```python
from build123d import *

# Parameters (mm, degrees)
F1_DEPTH = 30.1625
F2_DEPTH = 11.1633
F4_DEPTH = 19.05
F5_DEPTH = 19.05
F6_R     = 7.874
F7_R     = 5.08
F8_R     = 6.35
F9_DEPTH = 22.353


with BuildPart() as f1:
    # F0 (on Front) → F1 (new body, symmetric)
    with BuildSketch(Plane.XZ):
        Polygon((97.8408, -22.352), (117.2485877871, -22.352), (117.2485877871, 0), (91.8464, 0), align=None)
        Polygon((91.8464, -22.352), (91.8464, 0), (85.852, 0), align=None)
        Polygon((64.8810639977, -22.352), (91.8464, -22.352), (85.852, 0), (43.9732931554, 0), align=None)
        with BuildLine():
            Line((0, -22.352), (64.8810639977, -22.352))
            Line((64.8810639977, -22.352), (43.9732931554, 0))
            Line((43.9732931554, 0), (22.352, 0))
            ThreePointArc((22.352, 0), (15.8052507731, -15.8052507731), (0, -22.352))
        make_face()
        with BuildLine():
            ThreePointArc((22.352, 0), (-15.8052507731, 15.8052507731), (0, -22.352))
            Line((0, -22.352), (0, -12.7))
            ThreePointArc((0, -12.7), (-8.9802561211, 8.9802561211), (12.7, 0))
            Line((12.7, 0), (22.352, 0))
        make_face()
        Polygon((91.8464, -22.352), (97.8408, -22.352), (91.8464, 0), align=None)
        Polygon((194.2084, -22.352), (194.2084, 0), (150.0886, 0), (131.0386, 0), (117.2485877871, 0), (117.2485877871, -22.352), align=None)
        with BuildLine():
            Line((0, -12.7), (0, -22.352))
            ThreePointArc((0, -22.352), (15.8052507731, -15.8052507731), (22.352, 0))
            Line((22.352, 0), (12.7, 0))
            ThreePointArc((12.7, 0), (8.9802561211, -8.9802561211), (0, -12.7))
        make_face()
    extrude(amount=F1_DEPTH, both=True)

    # F0 (on Front) → F2 (cut, symmetric)
    with BuildSketch(Plane.XZ):
        with BuildLine():
            ThreePointArc((22.352, 0), (-15.8052507731, 15.8052507731), (0, -22.352))
            Line((0, -22.352), (0, -12.7))
            ThreePointArc((0, -12.7), (-8.9802561211, 8.9802561211), (12.7, 0))
            Line((12.7, 0), (22.352, 0))
        make_face()
        with BuildLine():
            Line((0, -12.7), (0, -22.352))
            ThreePointArc((0, -22.352), (15.8052507731, -15.8052507731), (22.352, 0))
            Line((22.352, 0), (12.7, 0))
            ThreePointArc((12.7, 0), (8.9802561211, -8.9802561211), (0, -12.7))
        make_face()
    extrude(amount=F2_DEPTH, both=True, mode=Mode.SUBTRACT)

    # F3 (on face) → F4 (cut)
    with BuildSketch(Plane.XZ.offset(30.1625)):
        Polygon((117.2485877871, -22.352), (117.2485877871, 0), (85.852, 0), (91.8464, -22.352), align=None)
    extrude(amount=-F4_DEPTH, mode=Mode.SUBTRACT)

    # F3 (on face) → F5 (join)
    with BuildSketch(Plane.XZ.offset(30.1625)):
        with BuildLine():
            ThreePointArc((131.0386, 34.798), (127.4654323074, 16.0825969798), (117.2485877871, 0))
            Line((117.2485877871, 0), (150.0886, 0))
            Line((150.0886, 0), (150.0886, 34.798))
            Line((150.0886, 34.798), (131.0386, 34.798))
        make_face()
    extrude(amount=-F5_DEPTH)

    # F6
    f6_edges = [f1.edges().sort_by_distance(p)[0] for p in [
        (194.2084, 0, 0),
    ]]
    fillet(f6_edges, radius=F6_R)

    # F7
    f7_edges = [f1.edges().sort_by_distance(p)[0] for p in [
        (150.0886, -20.6375, 34.798),
        (150.0886, -20.6375, 0),
        (22.352, 20.6629, 0),
        (22.352, -20.6629, 0),
    ]]
    fillet(f7_edges, radius=F7_R)

    # F8 (on face) → F9 (cut, through all)
    with BuildSketch(Plane.XY):
        with Locations((155.3464, 7.8105)):
            Circle(F8_R)
    extrude(amount=-F9_DEPTH, mode=Mode.SUBTRACT)


solid = f1.part
```
Design review of the part built by this model. Coordinates are the model's own, in mm. A direction names the side the tool comes from. Give positions to 0.01 mm unless a question says otherwise; leave off trailing zeros. Loops run counter-clockwise (first coordinate to the right, second up) from the corner with the lowest first, then second, coordinate; pieces in that order, holes last. Notation, with made-up numbers: M -25.5,89 L 33.5,89 A21 cw 33.5,105 Z; hole C 17,-30.75 d5. An arc over 180 degrees is marked long. Return JSON: item names as keys, results as strings. Group by question number.
Item 1: Mouldability with a two-part tool opening along Y and no side actions: class faces 5 (the flat face through (147, -30.162, 0)), 6 (the flat face through (13, 11.163, 0)), 7 (the flat face through (96, 0, -22.352)) as released by +Y, released by -Y, zero draft, split by the parting line, or undercut.
Item 2: We need section C-C (y = -6). Give the boundary of the cut face in (x, z).
Item 3: For probe 1 along Z at (x, y) = (0, -16); probe 2 along Y at (x, z) = (-3.5, 21); probe 3 along Z at (x, y) = (-0.5, 20.5), list the stretches that pass through material, from the lowest coordinate up.
Item 4: Tool access review of faces 1 (the flat face through (194.208, 0, -15)), 2 (the flat face through (117.249, -21, -11)), 3 (the cylindrical face through (23.8, -20.5, 1.1)), 4 (the flat face through (13, -11.163, 0)): name each direction out of +Z, -Z, +X, -X, +Y, -Y from which nothing blocks a thin tool from reaching the whole face with its end or side.
Item 5: Insertion check: pin 1 Ø20.5 at (x, y) = (155.35, 7.81) entering from +Z; pin 2 Ø5 at (y, z) = (9, 6) entering from +X; pin 3 Ø24.5 at (x, z) = (100.5, -13) entering from -Y; pin 4 Ø15 at (y, z) = (-19, -15.5) entering from -X. Each pin has a flat end and moves straight along its axis. Give the tip position at first contact, or say it passes through.
Item 6: We need section B-B (z = 19.5). Give the boundary of the cut face in (x, y), and give its area (3 significant figures).
Item 7: We need section A-A (y = -24.5). Give the boundary of the cut face in (x, z), and give its area (3 significant figures).
Item 8: We need section D-D (x = 71). Give the boundary of the cut face in (y, z).
Output:
{
 "1": {"face 5": "released by -Y", "face 6": "undercut", "face 7": "zero draft"},
 "2": {"outline": "M 0,-22.35 L 194.21,-22.35 L 194.21,-7.87 A7.87 ccw 186.33,0 L 22.35,0 A22.35 cw Z"},
 "3": {"probe 1": "z = -22.35 to -12.7, 12.7 to 22.35", "probe 2": "y = -30.16 to -11.16, 11.16 to 30.16", "probe 3": "z = -22.35 to -12.69, 12.69 to 22.35"},
 "4": {"face 1": "+Z, -Z, +X, +Y, -Y", "face 2": "+Z, -Z, -Y", "face 3": "+Z, +Y, -Y", "face 4": "+Z, -X"},
 "5": {"pin 1": "stops at z = 0", "pin 2": "stops at x = 21.84", "pin 3": "stops at y = -30.16", "pin 4": "stops at x = -20.87"},
 "6": {"outline": "M -10.93,-30.16 L 10.93,-30.16 L 10.93,-11.16 L -10.93,-11.16 Z; M -10.93,11.16 L 10.93,11.16 L 10.93,30.16 L -10.93,30.16 Z; M 128.68,-30.16 L 150.09,-30.16 L 150.09,-11.11 L 128.68,-11.11 Z", "area": "1,240 mm^2"},
 "7": {"outline": "M 0,-22.35 L 91.85,-22.35 L 85.85,0 L 26.96,0 A5.08 cw 21.97,4.14 A22.35 ccw long Z; M 117.25,-22.35 L 194.21,-22.35 L 194.21,-7.87 A7.87 ccw 186.33,0 L 155.17,0 A5.08 cw 150.09,5.08 L 150.09,29.72 A5.08 ccw 145.01,34.8 L 131.04,34.8 A50.8 cw 117.25,0 Z; hole C 0,0 d25.4", "area": "5,180 mm^2"},
 "8": {"outline": "M -30.16,-22.35 L 30.16,-22.35 L 30.16,0 L -30.16,0 Z"}
}
